Read the model definition and answer for the solid it produces. Units are mm, in the model's axes. Face numbers are marked on the shaded views. A direction names the side the tool comes from. Give positions to 0.01 mm unless a question says otherwise; leave off trailing zeros. Write each loop counter-clockwise with the first axis right and the second up, starting at its lowest first coordinate (ties: lowest second). Pieces come first, ordered by that corner, then holes. Notation, with made-up numbers: (45.25, -18) -> (86.25, -18) arc R23 cw to (86.25, -7) -> close; hole circle Ø3 at (70, -28). An arc over 180 degrees is marked (long way). Write item = value, one per line.
from build123d import *

# Parameters (mm, degrees)
SKETCH3_W           = 114
SKETCH3_H           = 164
BOSS_EXTRUDE2_DEPTH = 50
SKETCH4_W           = 100
SKETCH4_H           = 150
CUT_EXTRUDE2_DEPTH  = 45
SKETCH9_W           = 114
SKETCH9_H           = 5
CUT_EXTRUDE5_DEPTH  = 112.68258593
SKETCH10_W          = 114
SKETCH10_H          = 5
CUT_EXTRUDE6_DEPTH  = 112.68258593
SKETCH12_R          = 2.1
CUT_EXTRUDE8_DEPTH  = 20
SKETCH13_R          = 2.1
CUT_EXTRUDE9_DEPTH  = 20
SKETCH14_R          = 2.1
CUT_EXTRUDE10_DEPTH = 20
SKETCH15_W          = 5
SKETCH15_H          = 140
CUT_EXTRUDE11_DEPTH = 45
SKETCH16_R          = 3.5
BOSS_EXTRUDE3_DEPTH = 10
SKETCH17_R          = 1.75
CUT_EXTRUDE12_DEPTH = 8
SKETCH18_R          = 1.75
CUT_EXTRUDE13_DEPTH = 8
SKETCH19_W          = 9
SKETCH19_H          = 11
CUT_EXTRUDE14_DEPTH = 170.861708457
SKETCH21_R          = 3
CUT_EXTRUDE16_DEPTH = 170.861708457
SKETCH22_R          = 3
CUT_EXTRUDE17_DEPTH = 170.861708457


with BuildPart() as part:
    # Sketch3 → Boss-Extrude2 (new body)
    with BuildSketch(Plane(origin=(0, 0, 0), x_dir=(1, 0, 0), z_dir=(0, 1, 0))):
        Rectangle(SKETCH3_W, SKETCH3_H)
    extrude(amount=BOSS_EXTRUDE2_DEPTH)

    # Sketch4 → Cut-Extrude2 (cut)
    with BuildSketch(Plane(origin=(0, 50, 0), x_dir=(1, 0, 0), z_dir=(0, 1, 0))):
        Rectangle(SKETCH4_W, SKETCH4_H)
    extrude(amount=-CUT_EXTRUDE2_DEPTH, mode=Mode.SUBTRACT)

    # Sketch9 → Cut-Extrude5 (cut, through all)
    with BuildSketch(Plane(origin=(0, 50, 0), x_dir=(1, 0, 0), z_dir=(0, 1, 0))):
        with Locations((0, -79.5)):
            Rectangle(SKETCH9_W, SKETCH9_H)
    extrude(amount=-CUT_EXTRUDE5_DEPTH, mode=Mode.SUBTRACT)

    # Sketch10 → Cut-Extrude6 (cut, through all)
    with BuildSketch(Plane(origin=(0, 50, 0), x_dir=(1, 0, 0), z_dir=(0, 1, 0))):
        with Locations((0, 79.5)):
            Rectangle(SKETCH10_W, SKETCH10_H)
    extrude(amount=-CUT_EXTRUDE6_DEPTH, mode=Mode.SUBTRACT)

    # Sketch12 → Cut-Extrude8 (cut)
    with BuildSketch(Plane(origin=(0, 50, 0), x_dir=(1, 0, 0), z_dir=(0, 1, 0))):
        with Locations(Location((-53.236459808, -73.5, 0), (0, 0, 270))):
            Circle(SKETCH12_R)
    extrude(amount=-CUT_EXTRUDE8_DEPTH, mode=Mode.SUBTRACT)

    # Sketch13 → Cut-Extrude9 (cut)
    with BuildSketch(Plane(origin=(0, 50, 0), x_dir=(1, 0, 0), z_dir=(0, 1, 0))):
        with Locations(Location((53.5, -73.5, 0), (0, 0, 270))):
            Circle(SKETCH13_R)
    extrude(amount=-CUT_EXTRUDE9_DEPTH, mode=Mode.SUBTRACT)

    # Sketch14 → Cut-Extrude10 (cut)
    with BuildSketch(Plane(origin=(0, 50, 0), x_dir=(1, 0, 0), z_dir=(0, 1, 0))):
        with Locations(Location((53.5, 73.5, 0), (0, 0, 270))):
            Circle(SKETCH14_R)
        with Locations(Location((-53.5, 73.5, 0), (0, 0, 270))):
            Circle(SKETCH14_R)
    extrude(amount=-CUT_EXTRUDE10_DEPTH, mode=Mode.SUBTRACT)

    # Sketch15 → Cut-Extrude11 (cut)
    with BuildSketch(Plane(origin=(0, 50, 0), x_dir=(1, 0, 0), z_dir=(0, 1, 0))):
        with Locations((52.5, 0)):
            Rectangle(SKETCH15_W, SKETCH15_H)
    extrude(amount=-CUT_EXTRUDE11_DEPTH, mode=Mode.SUBTRACT)

    # Sketch16 → Boss-Extrude3 (add)
    with BuildSketch(Plane(origin=(0, 5, 0), x_dir=(1, 0, 0), z_dir=(0, 1, 0))):
        with Locations(Location((5.172888084, 43.030985647, 0), (0, 0, 90))):
            Circle(SKETCH16_R)
        with Locations(Location((6.475980518, -30.509718968, 0), (0, 0, 90))):
            Circle(SKETCH16_R)
    extrude(amount=BOSS_EXTRUDE3_DEPTH)

    # Sketch17 → Cut-Extrude12 (cut)
    with BuildSketch(Plane(origin=(0, 15, 0), x_dir=(1, 0, 0), z_dir=(0, 1, 0))):
        with Locations(Location((5.172888084, 43.030985647, 0), (0, 0, 270))):
            Circle(SKETCH17_R)
    extrude(amount=-CUT_EXTRUDE12_DEPTH, mode=Mode.SUBTRACT)

    # Sketch18 → Cut-Extrude13 (cut)
    with BuildSketch(Plane(origin=(0, 15, 0), x_dir=(1, 0, 0), z_dir=(0, 1, 0))):
        with Locations(Location((6.475980518, -30.509718968, 0), (0, 0, 270))):
            Circle(SKETCH18_R)
    extrude(amount=-CUT_EXTRUDE13_DEPTH, mode=Mode.SUBTRACT)

    # Sketch19 → Cut-Extrude14 (cut, through all)
    with BuildSketch(Plane(origin=(0, 0, 75), x_dir=(-1, 0, 0), z_dir=(0, 0, -1))):
        with Locations((44.222656572, 20.5)):
            Rectangle(SKETCH19_W, SKETCH19_H)
    extrude(amount=-CUT_EXTRUDE14_DEPTH, mode=Mode.SUBTRACT)

    # Sketch21 → Cut-Extrude16 (cut, through all)
    with BuildSketch(Plane.XY.offset(-75)):
        with Locations((42.25, 18)):
            Circle(SKETCH21_R)
    extrude(amount=-CUT_EXTRUDE16_DEPTH, mode=Mode.SUBTRACT)

    # Sketch22 → Cut-Extrude17 (cut, through all)
    with BuildSketch(Plane.XY.offset(-75)):
        with Locations((-42.95, 18)):
            Circle(SKETCH22_R)
    extrude(amount=-CUT_EXTRUDE17_DEPTH, mode=Mode.SUBTRACT)


solid = part.part
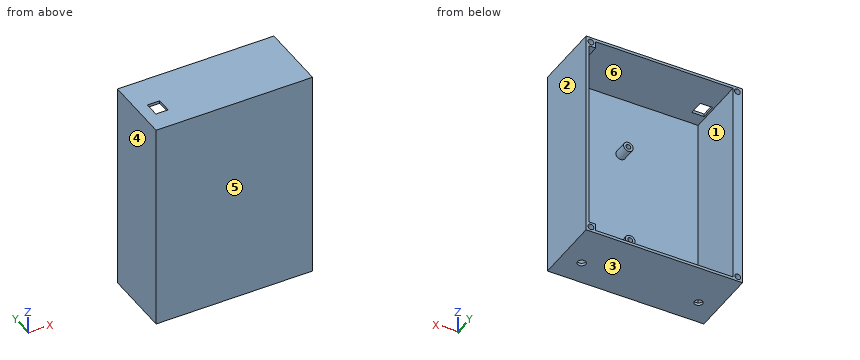
(1) Given P1, Ø4.5, axis at x = 5.17, z = -43.03, coming from the +Y side; P2, Ø4, axis at x = 53.5, z = -73.5, coming from the +Y side; P3, Ø1.5, axis at x = -42, y = 23, coming from the +Z side, each flat-ended and moving along its own axis, determine where each tip first touches the part or whether it passes through.
Checks:
P1 = 15
P2 = 30
P3 = -75
(2) The part is cut by section B-B on y = 18. Determine the outline of the cut face in (x, z), plus the area to 3 significant figures.
Checks:
outline = (-57, -77) -> (-45.95, -77) -> (-45.95, -75) -> (-50, -75) -> (-50, 75) -> (-48.72, 75) -> (-48.72, 77) -> (-57, 77) -> close; (-39.95, -77) -> (39.25, -77) -> (39.25, -75) -> (-39.95, -75) -> close; (-39.72, 75) -> (50, 75) -> (50, 70) -> (55, 70) -> (55, -70) -> (50, -70) -> (50, -75) -> (45.25, -75) -> (45.25, -77) -> (57, -77) -> (57, 77) -> (-39.72, 77) -> close
area = 1,810 mm²
(3) The part is cut by section C-C on x = -42.95. Determine the outline of the cut face in (y, z).
Checks:
outline = (0, -77) -> (15, -77) -> (15, -75) -> (5, -75) -> (5, 75) -> (15, 75) -> (15, 77) -> (0, 77) -> close; (21, -77) -> (50, -77) -> (50, -75) -> (21, -75) -> close; (26, 75) -> (50, 75) -> (50, 77) -> (26, 77) -> close
(4) The part is cut by section A-A on x = 42.25. Determine the outline of the cut face in (y, z), plus the area to 3 significant figures.
Checks:
outline = (0, -77) -> (15, -77) -> (15, -75) -> (5, -75) -> (5, 75) -> (50, 75) -> (50, 77) -> (0, 77) -> close; (21, -77) -> (50, -77) -> (50, -75) -> (21, -75) -> close
area = 938 mm²
(5) Consider L1, parallel to X at y = 40, z = -73.5; L2, parallel to Z at x = 9.5, y = 11; L3, parallel to X at y = 16, z = -3. Determine where each line is inside the solid, lowest interval first.
Checks:
L1 = -57 to -55.6, -51.4 to -50, 50 to 51.4, 55.6 to 57
L2 = -77 to -75, 28.75 to 32.27, 75 to 77
L3 = -57 to -50, 55 to 57
(6) The part is cut by section D-D on z = 49. Determine the outline of the cut face in (x, y).
Checks:
outline = (-57, 0) -> (57, 0) -> (57, 50) -> (55, 50) -> (55, 5) -> (-50, 5) -> (-50, 50) -> (-57, 50) -> close
(7) For a pull along X with two mould halves and no side action, classify the marked faces 1, 2, 3 and 4 as released by +X, released by -X, zero draft, split by the parting line, or undercut.
Checks:
face_1 = undercut
face_2 = released by +X
face_3 = zero draft
face_4 = released by -X
(8) A tool of negligible diameter and unlimited length cuts with its end or side. For the marked faces 5 and 6, from which of +Z, -Z, +X, -X, +Y, -Y can it reach the whole face along a straight path? Write none if from no direction.
Checks:
face_5 = +Z, -Z, +X, -X, -Y
face_6 = +Y
